Design review of the part shown in the three views and the two pictorial views. Dimensions are in mm from the part's minimum x, y and z. A direction names the side the tool comes from. Round coordinates to 2 decimals unless told otherwise and drop trailing zeros. Order: outer loops, then holes, each group sorted by start corner. A loop starts at its lowest first (then second) coordinate and runs counter-clockwise, first axis right, second up. Notation, with made-up numbers: M -34.5,50.25 L 7.5,50.25 A22 ccw 7.5,82.25 Z; hole C 21,52.25 d4. An arc over 180 degrees is marked long. Use a Markdown table: item, result. Add a question column.
(1) To check wall thickness, follow probe 1 along Y at (x, z) = (25.5, 5.75); probe 2 along Z at (x, y) = (13, 23.5); probe 3 along Z at (x, y) = (11.75, 22.5). State the ranges of each line that lie inside material, in increasing order. Write a range as from..to.
(2) Take a section at B-B (x = 15). Write out the cut boundary in (y, z), then the cut area to 3 significant figures.
(3) Take a section at D-D (x = 26.5). Write out the cut boundary in (y, z), then the cut area to 3 significant figures.
(4) Machinability: for the marked faces 1 and 2, which of the approach directions +Z, -Z, +X, -X, +Y, -Y give a long, thin tool a straight path to every point of the face, cutting with its end or side? Answer none if there is none.
(5) Take a section at C-C (y = 4.5). Write out the cut boundary in (x, z).
(6) For pin 1 (6 mm diameter, centred on y = 13.5, z = 17, fed in from -X); pin 2 (3 mm diameter, centred on x = 4, z = 17, fed in from -Y); pin 3 (5 mm diameter, centred on y = 12, z = 12, fed in from +X), all flat-tipped, find the tip position at first contact; note any pin that passes through.
(7) Take a section at A-A (z = 15). Write out the cut boundary in (x, y), then the cut area to 3 significant figures.
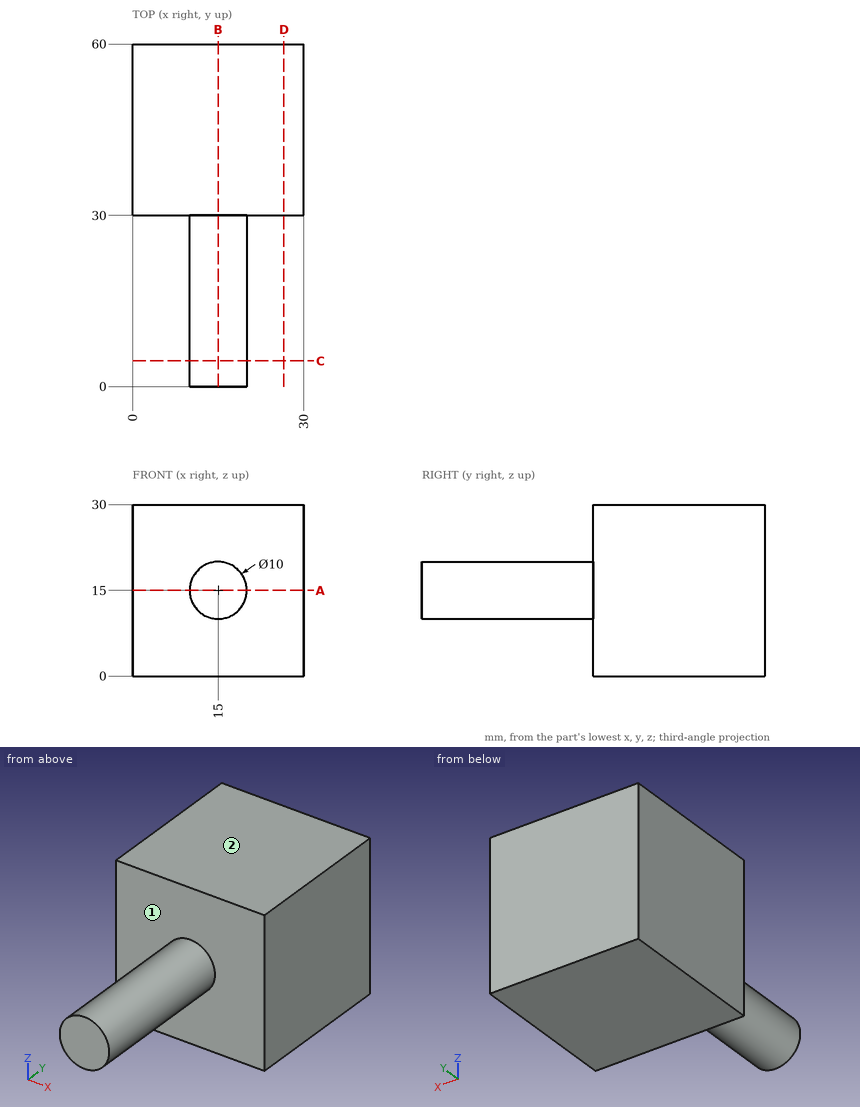
Verdict:
| question | item | result |
|---|---|---|
| 1 | probe 1 | y = 30..60 |
| 1 | probe 2 | z = 10.42..19.58 |
| 1 | probe 3 | z = 11.2..18.8 |
| 2 | outline | M 0,10 L 30,10 L 30,0 L 60,0 L 60,30 L 30,30 L 30,20 L 0,20 Z |
| 2 | area | 1,200 mm^2 |
| 3 | outline | M 30,0 L 60,0 L 60,30 L 30,30 Z |
| 3 | area | 900 mm^2 |
| 4 | face 1 | -Y |
| 4 | face 2 | +Z, +X, -X, +Y, -Y |
| 5 | outline | C 15,15 d10 |
| 6 | pin 1 | stops at x = 10 |
| 6 | pin 2 | stops at y = 30 |
| 6 | pin 3 | stops at x = 19.97 |
| 7 | outline | M 0,30 L 10,30 L 10,0 L 20,0 L 20,30 L 30,30 L 30,60 L 0,60 Z |
| 7 | area | 1,200 mm^2 |
